Read the model definition and answer for the solid it produces. Units are mm, in the model's axes. A direction names the side the tool comes from. Round coordinates to 2 decimals unless told otherwise and drop trailing zeros. Write each loop counter-clockwise with the first axis right and the second up, starting at its lowest first coordinate (ties: lowest second). Pieces come first, ordered by that corner, then holes. Notation, with made-up numbers: (85.5, 39.25) -> (142.5, 39.25) arc R8 cw to (142.5, 52.25) -> close; hole circle Ø5 at (-32, 27). An arc over 180 degrees is marked (long way). Return JSON: item names as keys, results as strings. Group by question number.
(1) A cutting plane is placed at C-C on z = -4. Give the vertices of the cut face in (x, y) (3 decimals), then the cut area to 3 significant figures.
(2) A cutting plane is placed at D-D on y = 89.5. Give the vertices of the cut face in (x, z).
(3) The mould has two halves that part along Z. Classify faces 1 (the flat face through (1, 47, 20.409)), 2 (the flat face through (-1, 100, 0)), 3 (the flat face through (-3.565, 86, 1)), 4 (the flat face through (1, 22.215, 0)): released by +Z, released by -Z, zero draft, split by the parting line, or undercut.
(4) Straight lines are drawn through the part: line 1 (Y direction, x = -3.5, z = -10.5) (3 decimals); line 2 (Z direction, x = 0.4, y = 86); line 3 (Y direction, x = 1.5, z = 16). For each, find the intervals that lie inside material, in ascending order.
(5) A cutting plane is placed at A-A on y = 78. Give the vertices of the cut face in (x, z).
(6) For faces 5 (the flat face through (-3.565, 18, 1)), 6 (the cylindrical face through (-4.654, 4.375, 11.203)), 7 (the cylindrical face through (3.98, 20.98, -8.39)), determine the directions among +Z, -Z, +X, -X, +Y, -Y from which every point of the face is accessible in a straight line to the end or side of a thin tool.
(7) A cutting plane is placed at B-B on x = 4. Give the vertices of the cut face in (y, z) (3 decimals), then the cut area to 3 significant figures.
(8) Given pin 1 (2.5 mm diameter, centred on y = 86, z = 9, fed in from +X); pin 2 (6.5 mm diameter, centred on y = 86, z = -8.72, fed in from -X); pin 3 (1.5 mm diameter, centred on x = -11.5, y = 16.5, fed in from -Z), each flat-ended and moving along its own axis, determine where each tip first touches the part or whether it passes through.
```python
from build123d import *
from build123d.topology import SkipClean

# Parameters (mm, degrees)
BOSS_EXTRUDE1_DEPTH = 100
SKETCH11_W          = 29.1
SKETCH11_H          = 75.5
CUT_EXTRUDE1_DEPTH  = 11.2
SKETCH13_R          = 4.4
CUT_EXTRUDE5_DEPTH  = 22.2
FILLET1_R           = 5
SKETCH14_W          = 29.1
SKETCH14_H          = 8.115
SKETCH14_R          = 2.75
SKETCH14_H_2        = 8.075
BOSS_EXTRUDE2_DEPTH = 0.72
SKETCH15_R          = 2.75
SKETCH15_R_2        = 1.25
BOSS_EXTRUDE3_DEPTH = 9.52
SKETCH16_R          = 2.5
CUT_EXTRUDE6_DEPTH  = 4
SKETCH17_W          = 29.764027379
SKETCH17_H          = 76.3
SKETCH17_W_2        = 28.964027379
SKETCH17_H_2        = 75.5
CUT_EXTRUDE7_DEPTH  = 44
SKETCH18_W          = 29.9
SKETCH18_H          = 60.11
SKETCH18_W_2        = 29.1
SKETCH18_H_2        = 59.31
CUT_EXTRUDE8_DEPTH  = 44
SKETCH19_W          = 29.764027379
SKETCH19_H          = 5.226630125
CUT_EXTRUDE9_DEPTH  = 44
SKETCH21_R          = 1
CUT_EXTRUDE10_DEPTH = 122.5
SKETCH22_R          = 1
CUT_EXTRUDE11_DEPTH = 10.5


with BuildPart() as part:
    # Sketch1 → Boss-Extrude1 (new body)
    with BuildSketch(Plane(origin=(0, 0, 0), x_dir=(1, 0, 0), z_dir=(0, 1, 0))):
        with BuildLine():
            Line((-4.0452326, 19.590813971), (5.9547674, 19.590813971))
            Line((5.9547674, 19.590813971), (5.9547674, -0.409186029))
            Line((5.9547674, -0.409186029), (5.9547674, -20.409186029))
            Line((5.9547674, -20.409186029), (-4.0452326, -20.409186029))
            ThreePointArc((-4.0452326, -20.409186029), (-11.116300412, -17.48025384), (-14.0452326, -10.409186029))
            Line((-14.0452326, -10.409186029), (-14.0452326, 9.590813971))
            ThreePointArc((-14.0452326, 9.590813971), (-11.116300412, 16.661881783), (-4.0452326, 19.590813971))
        make_face()
    extrude(amount=BOSS_EXTRUDE1_DEPTH)

    # Sketch11 → Cut-Extrude1 (cut)
    with BuildSketch(Plane.ZY.offset(14.0452326)):
        with Locations((0.409186029, 52.25)):
            Rectangle(SKETCH11_W, SKETCH11_H)
    extrude(amount=-CUT_EXTRUDE1_DEPTH, mode=Mode.SUBTRACT)

    # Sketch13 → Cut-Extrude5 (cut)
    with BuildSketch(Plane.ZY.offset(2.8452326)):
        with BuildLine():
            ThreePointArc((12.284186029, 86), (11.93014617, 87.349768499), (10.959186029, 88.351993835))
            ThreePointArc((10.959186029, 88.351993835), (9.534186029, 88.75), (8.109186029, 88.351993835))
            ThreePointArc((8.109186029, 88.351993835), (8.18441753, 83.604039858), (12.284186029, 86))
        make_face()
        with BuildLine():
            ThreePointArc((-5.965813971, 86), (-6.31985383, 87.349768499), (-7.290813971, 88.351993835))
            ThreePointArc((-7.290813971, 88.351993835), (-8.715813971, 88.75), (-10.140813971, 88.351993835))
            ThreePointArc((-10.140813971, 88.351993835), (-10.06558247, 83.604039858), (-5.965813971, 86))
        make_face()
        Polygon((4.229186029, 22.615), (14.959186029, 22.615), (14.959186029, 38.515), (14.959186029, 80.015), (14.959186029, 81.925), (4.229186029, 81.925), (2.559186029, 81.925), (-1.740813971, 81.925), (-3.410813971, 81.925), (-14.140813971, 81.925), (-14.140813971, 80.015), (-14.140813971, 38.515), (-14.140813971, 22.615), (-3.410813971, 22.615), (-1.740813971, 22.615), (2.559186029, 22.615), align=None)
        Polygon((12.984186029, 43.815), (12.984186029, 38.515), (12.984186029, 24.115), (-12.165813971, 24.115), (-12.165813971, 38.515), (-12.165813971, 43.815), align=None, mode=Mode.SUBTRACT)
        with BuildLine():
            ThreePointArc((7.989888554, 59.032180934), (6.768483101, 52.645011162), (6.359186029, 46.155))
            Line((6.359186029, 46.155), (-5.540813971, 46.155))
            ThreePointArc((-5.540813971, 46.155), (-5.950111044, 52.645011162), (-7.171516497, 59.032180934))
            ThreePointArc((-7.171516497, 59.032180934), (-7.78796768, 60.755318567), (-8.708121769, 62.337257826))
            ThreePointArc((-8.708121769, 62.337257826), (-9.536012183, 73.954242881), (0.409186029, 80.015))
            ThreePointArc((0.409186029, 80.015), (10.35438424, 73.954242881), (9.526493826, 62.337257826))
            ThreePointArc((9.526493826, 62.337257826), (8.606339737, 60.755318567), (7.989888554, 59.032180934))
        make_face(mode=Mode.SUBTRACT)
        with BuildLine():
            ThreePointArc((9.526493826, 62.337257826), (10.35438424, 73.954242881), (0.409186029, 80.015))
            ThreePointArc((0.409186029, 80.015), (-9.536012183, 73.954242881), (-8.708121769, 62.337257826))
            ThreePointArc((-8.708121769, 62.337257826), (-7.78796768, 60.755318567), (-7.171516497, 59.032180934))
            ThreePointArc((-7.171516497, 59.032180934), (-5.950111044, 52.645011162), (-5.540813971, 46.155))
            Line((-5.540813971, 46.155), (6.359186029, 46.155))
            ThreePointArc((6.359186029, 46.155), (6.768483101, 52.645011162), (7.989888554, 59.032180934))
            ThreePointArc((7.989888554, 59.032180934), (8.606339737, 60.755318567), (9.526493826, 62.337257826))
        make_face()
        with Locations((0.409186029, 68.825)):
            Circle(SKETCH13_R, mode=Mode.SUBTRACT)
        with Locations((0.409186029, 68.825)):
            Circle(SKETCH13_R)
        Polygon((12.984186029, 43.815), (12.984186029, 38.515), (12.984186029, 24.115), (-12.165813971, 24.115), (-12.165813971, 38.515), (-12.165813971, 43.815), align=None)
        with BuildLine():
            ThreePointArc((8.109186029, 16.148006165), (9.534186029, 15.75), (10.959186029, 16.148006165))
            ThreePointArc((10.959186029, 16.148006165), (11.93014617, 17.150231501), (12.284186029, 18.5))
            ThreePointArc((12.284186029, 18.5), (8.18441753, 20.895960142), (8.109186029, 16.148006165))
        make_face()
        with BuildLine():
            ThreePointArc((-10.140813971, 16.148006165), (-8.715813971, 15.75), (-7.290813971, 16.148006165))
            ThreePointArc((-7.290813971, 16.148006165), (-6.31985383, 17.150231501), (-5.965813971, 18.5))
            ThreePointArc((-5.965813971, 18.5), (-10.06558247, 20.895960142), (-10.140813971, 16.148006165))
        make_face()
    extrude(amount=-CUT_EXTRUDE5_DEPTH, mode=Mode.SUBTRACT)

    # Fillet1
    fillet1_edges = [part.edges().sort_by_distance(p)[0] for p in [
        (-11.116300412, 100, -16.661881783),
        (-14.0452326, 100, 0.409186029),
        (-11.116300412, 100, 17.48025384),
        (0.9547674, 100, 20.409186029),
        (0.9547674, 100, -19.590813971),
    ]]
    fillet(fillet1_edges, radius=FILLET1_R)

    # Sketch14 → Boss-Extrude2 (add)
    with SkipClean():  # the faces are left unmerged after this step: merging them gives an invalid solid
        with BuildSketch(Plane.ZY.offset(2.8452326)):
            with Locations((0.409186029, 18.5575)):
                Rectangle(SKETCH14_W, SKETCH14_H)
            with Locations((9.534186029, 18.5)):
                Circle(SKETCH14_R, mode=Mode.SUBTRACT)
            with Locations((-8.715813971, 18.5)):
                Circle(SKETCH14_R, mode=Mode.SUBTRACT)
            with Locations((0.409186029, 85.9625)):
                Rectangle(SKETCH14_W, SKETCH14_H_2)
            with Locations((9.534186029, 86)):
                Circle(SKETCH14_R, mode=Mode.SUBTRACT)
            with Locations((-8.715813971, 86)):
                Circle(SKETCH14_R, mode=Mode.SUBTRACT)
        extrude(amount=BOSS_EXTRUDE2_DEPTH)

    # Sketch15 → Boss-Extrude3 (add)
    with BuildSketch(Plane(origin=(5.9547674, 0, 0), x_dir=(0, 0, -1), z_dir=(1, 0, 0))):
        with Locations((8.715813971, 18.5)):
            Circle(SKETCH15_R)
        with Locations((8.715813971, 18.5)):
            Circle(SKETCH15_R_2, mode=Mode.SUBTRACT)
        with Locations((-9.534186029, 18.5)):
            Circle(SKETCH15_R)
        with Locations((-9.534186029, 18.5)):
            Circle(SKETCH15_R_2, mode=Mode.SUBTRACT)
        with Locations((8.715813971, 86)):
            Circle(SKETCH15_R)
        with Locations((8.715813971, 86)):
            Circle(SKETCH15_R_2, mode=Mode.SUBTRACT)
        with Locations((-9.534186029, 86)):
            Circle(SKETCH15_R)
        with Locations((-9.534186029, 86)):
            Circle(SKETCH15_R_2, mode=Mode.SUBTRACT)
    extrude(amount=-BOSS_EXTRUDE3_DEPTH)

    # Sketch16 → Cut-Extrude6 (cut)
    with BuildSketch(Plane(origin=(5.9547674, 0, 0), x_dir=(0, 0, -1), z_dir=(1, 0, 0))):
        with Locations((-9.534186029, 18.5)):
            Circle(SKETCH16_R)
        with Locations((8.715813971, 18.5)):
            Circle(SKETCH16_R)
        with Locations((-9.534186029, 86)):
            Circle(SKETCH16_R)
        with Locations((8.715813971, 86)):
            Circle(SKETCH16_R)
    extrude(amount=-CUT_EXTRUDE6_DEPTH, mode=Mode.SUBTRACT)

    # Sketch17 → Cut-Extrude7 (cut)
    with BuildSketch(Plane.ZY.offset(3.5652326)):
        with Locations((0.341199719, 52.25)):
            Rectangle(SKETCH17_W, SKETCH17_H)
        with Locations((0.341199719, 52.25)):
            Rectangle(SKETCH17_W_2, SKETCH17_H_2, mode=Mode.SUBTRACT)
    extrude(amount=CUT_EXTRUDE7_DEPTH, mode=Mode.SUBTRACT)

    # Sketch18 → Cut-Extrude8 (cut)
    with BuildSketch(Plane.ZY.offset(3.5652326)):
        with Locations((0.409186029, 52.27)):
            Rectangle(SKETCH18_W, SKETCH18_H)
        with Locations((0.409186029, 52.27)):
            Rectangle(SKETCH18_W_2, SKETCH18_H_2, mode=Mode.SUBTRACT)
    extrude(amount=-CUT_EXTRUDE8_DEPTH, mode=Mode.SUBTRACT)

    # Sketch19 → Cut-Extrude9 (cut)
    with BuildSketch(Plane.ZY.offset(14.0452326)):
        with Locations((0.341199719, 11.486684938)):
            Rectangle(SKETCH19_W, SKETCH19_H)
    extrude(amount=-CUT_EXTRUDE9_DEPTH, mode=Mode.SUBTRACT)

    # Sketch21 → Cut-Extrude10 (cut)
    with BuildSketch(Plane(origin=(0, 0, -19.590813971), x_dir=(-1, 0, 0), z_dir=(0, 0, -1))):
        with Locations((-0.9547674, 71.936684938)):
            Circle(SKETCH21_R)
        with Locations((-0.9547674, 31.936684938)):
            Circle(SKETCH21_R)
    extrude(amount=-CUT_EXTRUDE10_DEPTH, mode=Mode.SUBTRACT)

    # Sketch22 → Cut-Extrude11 (cut)
    with BuildSketch(Plane.XZ):
        with Locations(Location((-4.0452326, -9.590813971, 0), (0, 0, 270))):
            Circle(SKETCH22_R)
        with Locations(Location((-4.0452326, 10.409186029, 0), (0, 0, 270))):
            Circle(SKETCH22_R)
    extrude(amount=-CUT_EXTRUDE11_DEPTH, mode=Mode.SUBTRACT)


solid = part.part
```
Checks:
{
 "1": {"outline": "(-14.045, 0) -> (5.955, 0) -> (5.955, 8.873) -> (-14.045, 8.873) -> close; (-14.045, 90.4) -> (-3.565, 90.4) -> (-3.565, 82.325) -> (5.955, 82.325) -> (5.955, 100) -> (-9.045, 100) arc R5 ccw to (-14.045, 95) -> close; (-3.565, 14.1) -> (5.955, 14.1) -> (5.955, 22.215) -> (-3.565, 22.215) -> close", "area": "518 mm^2"},
 "2": {"outline": "(-12.81, 15.22) -> (-3.57, 15.22) -> (-3.57, -14.54) -> (-12.73, -14.54) arc R10 ccw to (-4.05, -19.59) -> (5.95, -19.59) -> (5.95, 20.41) -> (-4.05, 20.41) arc R10 ccw to start"},
 "3": {"face 1": "released by +Z", "face 2": "zero draft", "face 3": "undercut", "face 4": "undercut"},
 "4": {"line 1": "y = 0 to 8.873, 14.1 to 22.215, 82.325 to 100", "line 2": "z = -19.59 to -9.97, -7.47 to 8.28, 10.78 to 20.41", "line 3": "y = 0 to 31.1, 32.77 to 71.1, 72.77 to 99.96"},
 "5": {"outline": "(-12.81, 15.22) -> (-3.57, 15.22) -> (-3.57, 15.36) -> (5.95, 15.36) -> (5.95, 20.41) -> (-4.05, 20.41) arc R10 ccw to start; (-12.73, -14.54) arc R10 ccw to (-4.05, -19.59) -> (5.95, -19.59) -> (5.95, -14.54) -> close"},
 "6": {"face 5": "-X", "face 6": "-Y", "face 7": "+X"},
 "7": {"outline": "(0, -19.591) -> (95, -19.591) arc R5 ccw to (100, -14.591) -> (100, 15.409) arc R5 ccw to (95, 20.409) -> (0, 20.409) -> close; hole (8.873, -14.541) -> (14.1, -14.541) -> (14.1, 15.223) -> (8.873, 15.223) -> close; hole circle Ø5 at (18.5, -8.716); hole circle Ø5 at (18.5, 9.534); hole (22.215, -14.541) -> (82.325, -14.541) -> (82.325, 15.359) -> (22.215, 15.359) -> close; hole circle Ø5 at (86, -8.716); hole circle Ø5 at (86, 9.534)", "area": "1,960 mm^2"},
 "8": {"pin 1": "stops at x = 1.95", "pin 2": "stops at x = -3.57", "pin 3": "stops at z = -17.01"}
}
